```python
from build123d import *

# Parameters (mm, degrees)
SKETCH1_W                    = 114.3
SKETCH1_H                    = 101.6
BOSS_EXTRUDE1_DEPTH          = 6.35
FILLET1_R                    = 6.35
F_3_8_0_375_DIAMETER_HOLE1_D = 9.525


with BuildPart() as part:
    # Sketch1 → Boss-Extrude1 (new body)
    with BuildSketch(Plane(origin=(0, 0, 0), x_dir=(1, 0, 0), z_dir=(0, 1, 0))):
        Rectangle(SKETCH1_W, SKETCH1_H)
    extrude(amount=BOSS_EXTRUDE1_DEPTH)

    # Fillet1
    fillet1_edges = [part.edges().sort_by_distance(p)[0] for p in [
        (-57.15, 3.175, -50.8),
        (57.15, 3.175, -50.8),
        (57.15, 3.175, 50.8),
        (-57.15, 3.175, 50.8),
    ]]
    fillet(fillet1_edges, radius=FILLET1_R)

    # 3/8 (0.375) Diameter Hole1 (through all)
    with Locations(Plane(origin=(46.0375, 6.35, 38.1), x_dir=(0, 0, 1), z_dir=(0, 1, 0))):
        with Locations((0, 0), (0, -92.075), (-76.2, -92.075), (-76.2, 0)):
            Hole(F_3_8_0_375_DIAMETER_HOLE1_D / 2)


solid = part.part
```
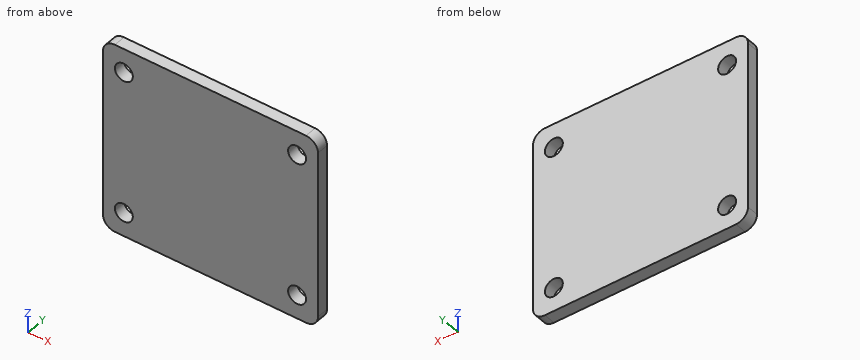
CAD build for the part. Positions are in the model's coordinates, mm. Round coordinates to 2 decimals unless told otherwise and drop trailing zeros. Order: outer loops, then holes, each group sorted by start corner. A loop starts at its lowest first (then second) coordinate and runs counter-clockwise, first axis right, second up. Notation, with made-up numbers: (3, 24.25) -> (7, 24.25) arc R11 cw to (7, 33.25) -> close; hole circle Ø3 at (88.25, 60.25). An arc over 180 degrees is marked (long way). One line per question, with ' | ' between items.
Q1. Drop a flat-ended pin along its axis: pin 1 (5.5 mm diameter, centred on x = -46.04, z = 38.1, fed in from +Y). Give the stop position or say it passes through.
Completed:
pin 1: passes through
Q2. Probe probe 1 along X at (y, z) = (0.5, -38); probe 2 along X at (y, z) = (2.25, 35); probe 3 along Z at (x, y) = (-49.5, 3). List the from-to ranges inside material, lowest first.
Completed:
probe 1: x = -57.15 to -50.8, -41.28 to 41.28, 50.8 to 57.15 | probe 2: x = -57.15 to -49.65, -42.42 to 42.42, 49.65 to 57.15 | probe 3: z = -50.8 to -41.37, -34.83 to 34.83, 41.37 to 50.8
Q3. Slice it at B-B (y = 4). Give the number of separate pieces and of enclosed holes in the cut face, then the cut area to 3 significant figures.
Completed:
separate pieces: 1 | enclosed holes: 4 | area: 11,300 mm^2
Q4. Slice it at C-C (x = 44). Write the cut outline in (y, z).
Completed:
outline: (0, -50.8) -> (6.35, -50.8) -> (6.35, -42.4) -> (0, -42.4) -> close; (0, -33.8) -> (6.35, -33.8) -> (6.35, 33.8) -> (0, 33.8) -> close; (0, 42.4) -> (6.35, 42.4) -> (6.35, 50.8) -> (0, 50.8) -> close
Q5. Slice it at A-A (z = 38.1). Write the cut outline in (x, y) (3 decimals).
Completed:
outline: (-57.15, 0) -> (-50.8, 0) -> (-50.8, 6.35) -> (-57.15, 6.35) -> close; (-41.275, 0) -> (41.275, 0) -> (41.275, 6.35) -> (-41.275, 6.35) -> close; (50.8, 0) -> (57.15, 0) -> (57.15, 6.35) -> (50.8, 6.35) -> close
